from build123d import *

# Parameters (mm, degrees)
SKETCH_1_W          = 135
SKETCH_1_H          = 75
SKETCH_1_R          = 10.5
SKETCH_1_W_2        = 87
SKETCH_1_H_2        = 57
EXTRUDE_1_DEPTH     = 3
SKETCH_5_R          = 15
SKETCH_4_R          = 12.5
CUT_EXTRUDE_1_REACH = 171.52
SKETCH_5_93_R       = 10.5


with BuildPart() as part:
    # 草图1 → 凸台-拉伸1 (new body)
    with BuildSketch(Plane(origin=(0, 0, 902.944534426), x_dir=(-1, 0, 0), z_dir=(0, 0, -1))):
        with Locations((-85.5, 34.5)):
            Rectangle(SKETCH_1_W, SKETCH_1_H)
        with Locations((-33, 34.5)):
            Circle(SKETCH_1_R, mode=Mode.SUBTRACT)
        with Locations((-93, 34.5)):
            Rectangle(SKETCH_1_W_2, SKETCH_1_H_2, mode=Mode.SUBTRACT)
    extrude(amount=EXTRUDE_1_DEPTH)

    # 草图5 → 放样4 section 0
    with BuildSketch(Plane(origin=(0, 0, 899.944534426), x_dir=(-1, 0, 0), z_dir=(0, 0, -1))):
        with Locations((-33, 34.5)):
            Circle(SKETCH_5_R)
    # 草图4 → 放样4 section 1
    with BuildSketch(Plane.XY.offset(887.944534426)):
        with Locations((33, 34.5)):
            Circle(SKETCH_4_R)
    loft()

    # 草图5<93> → 切除-拉伸1 (cut, up to next)
    with BuildSketch(Plane(origin=(0, 0, 899.944534426), x_dir=(-1, 0, 0), z_dir=(0, 0, -1)), mode=Mode.PRIVATE) as cut_extrude_1_sk1:
        with Locations(Location((-33, 34.5, 0), (0, 0, 180))):
            Circle(SKETCH_5_93_R)
    cut_extrude_1_tool1 = extrude(cut_extrude_1_sk1.sketch, amount=CUT_EXTRUDE_1_REACH, mode=Mode.PRIVATE) & part.part
    add(cut_extrude_1_tool1.solids().sort_by_distance((33, 34.5, 899.944534))[0], mode=Mode.SUBTRACT)


solid = part.part
Build history of the part. All positions in model axes, mm. A direction names the side the tool comes from. Give positions to 0.01 mm unless a question says otherwise; leave off trailing zeros. Loops run counter-clockwise (first coordinate to the right, second up) from the corner with the lowest first, then second, coordinate; pieces in that order, holes last. Notation, with made-up numbers: (-24.5, 24) - (29.5, 24) arc R19 cw to (29.5, 49) - close; hole circle Ø5 at (76.5, -15). An arc over 180 degrees is marked (long way). Write item = value, one per line. Start each with the question number.
1) Band-saw the part on B-B on x = 117. Give the cut face in (y, z).
2) Tool access for faces 1 (the flat face through (153, 34, 901)), 2 (the flat face through (94, 63, 901)): list every direction of +Z, -Z, +X, -X, +Y, -Y with a clear straight run to the whole face (end or side of a thin tool).
3) Probe probe 1 along Z at (x, y) = (74, 69); probe 2 along Y at (x, z) = (26, 893.75); probe 3 along Y at (x, z) = (33, 899.5). List the from-to ranges inside material, lowest first. Write a range as from..to.
4) Band-saw the part on C-C on z = 891. Give the cut face in (x, y).
5) Band-saw the part on A-A on y = 17.5. Give the cut face in (x, z), plus the area to 3 significant figures.
6) Pull direction X, two halves, no side cores. Call faces 3 (the flat face through (94, 6, 901)), 4 (the flat face through (86, -3, 901)), 5 (the flat face through (18, 34, 901)): +X half, -X half, draft (parallel to the pull), parting line (faces both ways), or undercut.
7) Drop flat-ended pins along their axis: pin 1 Ø3 at (y, z) = (33, 897.5) entering from +X; pin 2 Ø8 at (y, z) = (44.5, 889.5) entering from +X; pin 3 Ø3 at (y, z) = (41, 891.5) entering from +X. Give the stop position or say it passes through.
Final values:
q1.outline = (-3, 899.94) - (6, 899.94) - (6, 902.94) - (-3, 902.94) - close; (63, 899.94) - (72, 899.94) - (72, 902.94) - (63, 902.94) - close
q2.face_1 = +Z, -Z, +X, +Y, -Y
q2.face_2 = +Z, -Z
q3.probe_1 = 899.94..902.94
q3.probe_2 = 22.71..26.67, 42.33..46.29
q3.probe_3 = 19.59..24, 45..49.41
q4.outline = circle Ø26.27 at (33, 34.5); hole circle Ø21 at (33, 34.5)
q5.outline = (18, 899.94) - (49.5, 899.94) - (49.5, 902.94) - (18, 902.94) - close; (136.5, 899.94) - (153, 899.94) - (153, 902.94) - (136.5, 902.94) - close
q5.area = 144 mm²
q6.face_3 = undercut
q6.face_4 = draft
q6.face_5 = -X half
q7.pin_1 = 47.75
q7.pin_2 = 44.53
q7.pin_3 = 45.35
